The figure shows three views and two pictorial views of one solid part (mm, origin at its lowest corner). Answer the questions. A direction names the side the tool comes from. Coordinates: 2 decimals unless noted, no trailing zeros. Order: outer loops, then holes, each group sorted by start corner. A loop starts at its lowest first (then second) coordinate and runs counter-clockwise, first axis right, second up. Notation, with made-up numbers: (64.5, 6) -> (105.5, 6) arc R24 cw to (105.5, 19) -> close; hole circle Ø3 at (-19.75, 70). An arc over 180 degrees is marked (long way). Write item = value, one per line. Start each with the question number.
Q1. The part is cut by section C-C, the plane x = 55. Determine the outline of the cut face in (y, z), plus the area to 3 significant figures.
Q2. Flat-ended cylindrical pins translate along their axes: pin 1 (5 mm diameter, centred on x = 12.5, z = 3, fed in from +Y); pin 2 (2.5 mm diameter, centred on x = 4, y = 10, fed in from -Z); pin 3 (1.2 mm diameter, centred on x = 5, z = 3.5, fed in from +Y). Find the tip coordinate at first contact, or state that the pin passes through.
Q3. The part is cut by section B-B, the plane z = 9. Determine the outline of the cut face in (x, y), plus the area to 3 significant figures.
Q4. For a pull along X with two mould halves and no side action, classify the marked faces 1, 2 and 3 as +X half, -X half, draft (parallel to the pull), parting line (faces both ways), or undercut.
Q5. Straight lines are drawn through the part: L1, parallel to Y at x = 4, z = 4.5; L2, parallel to Y at x = 56, z = 6; L3, parallel to X at y = 39, z = 7.75. For each, find the intervals that lie inside material, in ascending order. Write a range as from..to.
Q6. Which of the six approach directions +Z, -Z, +X, -X, +Y, -Y give full straight-line access (tool end or side, diameter ignored) to the marked faces 4 and 5?
Q7. The part is cut by section A-A, the plane y = 36.5. Determine the outline of the cut face in (x, z), plus the area to 3 significant figures.
Q8. The part is cut by section D-D, the plane y = 10. Determine the outline of the cut face in (x, z).
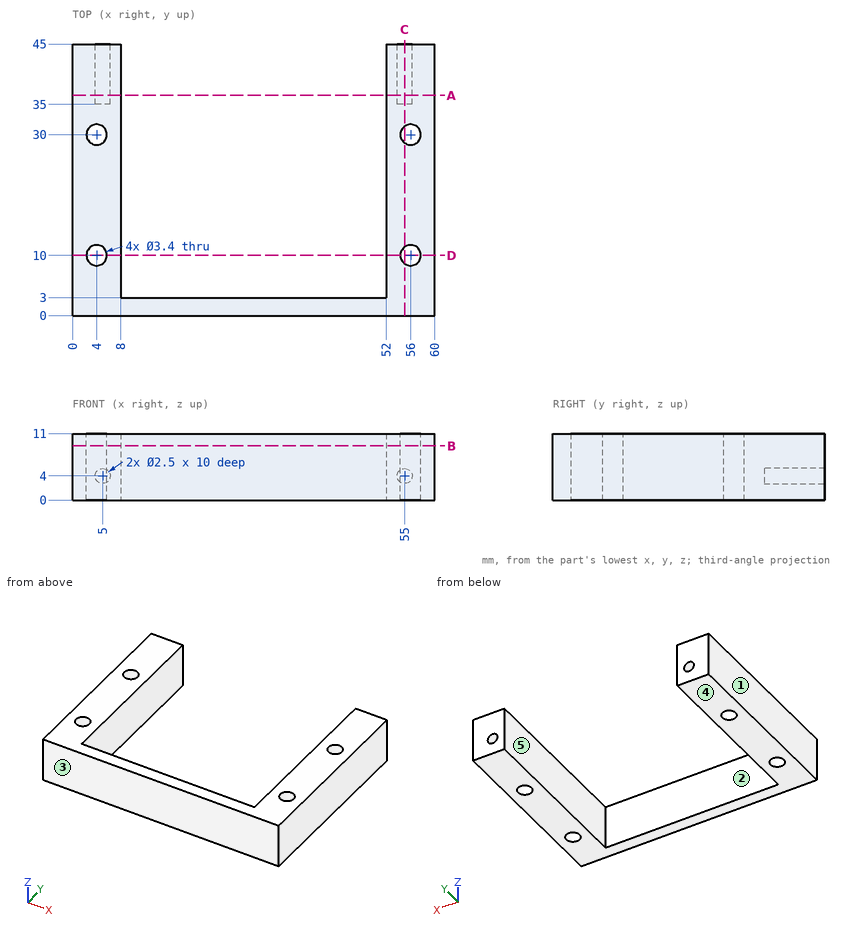
Model answer:
q1.outline = (0, 0) -> (8.63, 0) -> (8.63, 11) -> (0, 11) -> close; (11.37, 0) -> (28.63, 0) -> (28.63, 11) -> (11.37, 11) -> close; (31.37, 0) -> (45, 0) -> (45, 2.75) -> (35, 2.75) -> (35, 5.25) -> (45, 5.25) -> (45, 11) -> (31.37, 11) -> close
q1.area = 410 mm2
q2.pin_1 = 3
q2.pin_2 = through
q2.pin_3 = 35
q3.outline = (0, 0) -> (60, 0) -> (60, 45) -> (52, 45) -> (52, 3) -> (8, 3) -> (8, 45) -> (0, 45) -> close; hole circle Ø3.4 at (4, 10); hole circle Ø3.4 at (4, 30); hole circle Ø3.4 at (56, 10); hole circle Ø3.4 at (56, 30)
q3.area = 816 mm2
q4.face_1 = -X half
q4.face_2 = undercut
q4.face_3 = draft
q5.L1 = 0..8.3, 11.7..28.3, 31.7..35
q5.L2 = 0..8.3, 11.7..28.3, 31.7..45
q5.L3 = 0..8, 52..60
q6.face_4 = -Z, +X, -X, +Y, -Y
q6.face_5 = +Z, -Z, +Y
q7.outline = (0, 0) -> (8, 0) -> (8, 11) -> (0, 11) -> close; (52, 0) -> (60, 0) -> (60, 11) -> (52, 11) -> close; hole circle Ø2.5 at (5, 4); hole circle Ø2.5 at (55, 4)
q7.area = 166 mm2
q8.outline = (0, 0) -> (2.3, 0) -> (2.3, 11) -> (0, 11) -> close; (5.7, 0) -> (8, 0) -> (8, 11) -> (5.7, 11) -> close; (52, 0) -> (54.3, 0) -> (54.3, 11) -> (52, 11) -> close; (57.7, 0) -> (60, 0) -> (60, 11) -> (57.7, 11) -> close
